from build123d import *

# Parameters (mm, degrees)
F0_R     = 12.446
F0_R_2   = 6.35
F1_DEPTH = 41.91
F2_R     = 15.875
F2_R_2   = 6.35
F3_DEPTH = 3.175
F5_R     = 0.9525
F6_DEPTH = 41.276


with BuildPart() as f1:
    # F0 (on Front) → F1 (new body)
    with BuildSketch(Plane.XZ):
        Circle(F0_R)
        Circle(F0_R_2, mode=Mode.SUBTRACT)
    extrude(amount=F1_DEPTH)

    # F2 (on Front) → F3 (join)
    with BuildSketch(Plane.XZ):
        Circle(F2_R)
        Circle(F2_R_2, mode=Mode.SUBTRACT)
    extrude(amount=-F3_DEPTH)

    # F5 (on offset) → F6 (cut, through all)
    with BuildSketch(Plane.XY.offset(25.4)):
        with Locations((0, -40.005)):
            Circle(F5_R)
    extrude(amount=-F6_DEPTH, mode=Mode.SUBTRACT)


solid = f1.part
Verification items for the finished model (mm, model axes). A direction names the side the tool comes from. Coordinates: 2 decimals unless noted, no trailing zeros. Write each loop counter-clockwise with the first axis right and the second up, starting at its lowest first coordinate (ties: lowest second). Pieces come first, ordered by that corner, then holes. Notation, with made-up numbers: (37, 64) -> (77, 64) arc R19 cw to (77, 90) -> close; hole circle Ø1 at (82, 21). An arc over 180 degrees is marked (long way). One line per item, written item: value. Start each with the question number.
Q1. Thickness scan on L1, parallel to Y at x = 0, z = 8 (1 decimal); L2, parallel to Z at x = 0, y = -14; L3, parallel to Y at x = 12, z = 6 (3 decimals). Record the ranges inside material, lowest first. Write a range as from..to.
Q2. Cross-section at A-A on x = 0. State how many separate pieces and enclosed holes the cut face has, and give its area (3 significant figures).
Q3. Go/stop test with flat-tipped pins: P1, Ø5, axis at x = -4, y = -25.5, coming from the +Z side; P2, Ø4, axis at y = -11, z = -6, coming from the -X side; P3, Ø1, axis at y = -22, z = -2, coming from the -X side; P4, Ø12, axis at x = -12, z = 3.5, coming from the -Y side. Record where each tip stops, or that it passes through.
Q4. Cross-section at B-B on z = 0. Enter the section's corners in (x, y) (3 decimals), and give its area (3 significant figures).
Q5. Cross-section at C-C on x = 11. Enter the section's corners in (y, z) (3 decimals).
Q6. Cross-section at D-D on y = -21. Enter the section's corners in (x, z).
Q7. Access from +Z, -Z, +X, -X, +Y, -Y to the whole of each face (thin tool, end or side, straight path). Record for faces 1 (the flat face through (7, 3.175, 0)), 2 (the flat face through (7, 0, -11)).
Q8. Mould release check, pull along Z, two halves, no side actions. Record for faces 3 (the cylindrical face through (-3.441, 1.565, -15.497)), 4 (the cylindrical face through (-1.38, -19.68, -6.2)), 5 (the flat face through (-6, -41.91, 3)): pulls with the +Z half, pulls with the -Z half, needs draft (parallel to the pull), parting line crosses it, or undercut.
Checked values:
1. L1: y = -41.9..-41, -39.1..3.2
1. L2: z = -12.45..-6.35, 6.35..12.45
1. L3: y = 0..3.175
2. separate pieces: 4
2. enclosed holes: 0
2. area: 548 mm²
3. P1: stops at z = 12.36
3. P2: stops at x = -11.79
3. P3: stops at x = -12.36
3. P4: stops at y = -41.91
4. outline: (-15.875, 0) -> (-12.446, 0) -> (-12.446, -41.91) -> (-6.35, -41.91) -> (-6.35, 3.175) -> (-15.875, 3.175) -> close; (6.35, -41.91) -> (12.446, -41.91) -> (12.446, 0) -> (15.875, 0) -> (15.875, 3.175) -> (6.35, 3.175) -> close
4. area: 571 mm²
5. outline: (-41.91, -5.823) -> (0, -5.823) -> (0, -11.446) -> (3.175, -11.446) -> (3.175, 11.446) -> (0, 11.446) -> (0, 5.823) -> (-41.91, 5.823) -> close
6. outline: circle Ø24.89 at (0, 0); hole circle Ø12.7 at (0, 0)
7. face 1: +Z, -Z, +X, -X, +Y
7. face 2: -Y
8. face 3: parting line crosses it
8. face 4: undercut
8. face 5: needs draft
